Geometry: final body of the model. Coordinates: model frame, mm. A direction names the side the tool comes from. Give positions to 0.01 mm unless a question says otherwise; leave off trailing zeros. Loops run counter-clockwise (first coordinate to the right, second up) from the corner with the lowest first, then second, coordinate; pieces in that order, holes last. Notation, with made-up numbers: (56, 46) -> (67, 46) arc R25 cw to (67, 64) -> close; hole circle Ø7 at (31.25, 61.25). An arc over 180 degrees is marked (long way). Answer in a Markdown table with one row per item. Add a question column.
1) Access query for faces 1 (the cylindrical face through (0.32, 21.08, -13.44)), 2 (the flat face through (-9, -70, 0)), 3 (the flat face through (-20, -77, 0)), 4 (the flat face through (-15, 0, 55)), 5 (the flat face through (0, 18, 58)). Directions: +Z, -Z, +X, -X, +Y, -Y. A direction counts if a zero-diameter tool reaches every point of the face in a straight line with its end or side. Return the directions, or none.
2) Draft query along Z for faces 6 (the flat face through (-23, 5.9, 11.5)), 7 (the flat face through (15, 0, 55)), 8 (the cylindrical face through (37.13, -134.84, -12.92)). Return one class per face: +Z half, -Z half, draft (parallel to the pull), parting line (faces both ways), or undercut.
3) First-contact query: P1, Ø3, axis at x = -10, z = 22.5, coming from the +Y side; P2, Ø11, axis at y = -4.5, z = 44.5, coming from the -X side; P3, Ø10, axis at x = 33, y = -93, coming from the +Z side; P4, Ø19, axis at y = -110, z = 0, coming from the -X side. Flat tips, straight axial feed; report the tip coordinate or a pass-through.
4) Line query: line 1 (X direction, y = -111.5, z = 19); line 2 (Z direction, x = -10.25, y = -110); line 3 (Z direction, x = -8, y = -15). Output: solid intervals per line, ascending. Write a range as from..to.
5) Section query A-A (z = 0). Give the number of separate pieces and of enclosed holes in the cut face, plus the area to 3 significant figures.
6) Section query B-B (x = -2). Return the cut outline in (y, z).
7) Section query D-D (z = 90.5). Return the cut outline in (x, y), plus the area to 3 significant figures.
8) Section query C-C (y = -110). Return the cut outline in (x, z).
```python
from build123d import *

# Parameters (mm, degrees)
SKETCH1_R               = 25
SKETCH1_R_2             = 12.5
BOSS_EXTRUDE1_DEPTH     = 23
BOSS_EXTRUDE3_START     = 20
BOSS_EXTRUDE3_DEPTH     = 18
SKETCH5_R               = 28
SKETCH5_R_2             = 16
BOSS_EXTRUDE4_DEPTH     = 35
BOSS_EXTRUDE5_DEPTH     = 31
CUT_EXTRUDE2_DEPTH      = 155.819249449
CUT_EXTRUDE2_DEPTH_BACK = 155.819249449
SKETCH6_W               = 34
SKETCH6_H               = 70
SKETCH8_R               = 18
SKETCH8_R_2             = 7.5
BOSS_EXTRUDE6_DEPTH     = 24
BOSS_EXTRUDE7_DEPTH     = 21
BOSS_EXTRUDE8_DEPTH     = 9
CUT_EXTRUDE4_DEPTH      = 193.512337267
CUT_EXTRUDE4_DEPTH_BACK = 193.512337267
SKETCH10_W              = 18
SKETCH10_H              = 50


with BuildPart() as part:
    # Sketch1 → Boss-Extrude1 (new, symmetric)
    with BuildSketch(Plane(origin=(0, 0, 0), x_dir=(0, 0, -1), z_dir=(1, 0, 0))):
        Circle(SKETCH1_R)
        Circle(SKETCH1_R_2, mode=Mode.SUBTRACT)
    extrude(amount=BOSS_EXTRUDE1_DEPTH, both=True)

    # Sketch4 → Boss-Extrude3 (add)
    with BuildSketch(Plane(origin=(0, 0, 0), x_dir=(0, 0, -1), z_dir=(1, 0, 0)).offset(BOSS_EXTRUDE3_START)):
        with BuildLine():
            Line((-25, 0), (-25, -70))
            Line((-25, -70), (25, -70))
            Line((25, -70), (25, 0))
            ThreePointArc((25, 0), (0, -25), (-25, 0))
        make_face()
    extrude(amount=-BOSS_EXTRUDE3_DEPTH)



with BuildPart() as body_2:
    # Sketch5 → Boss-Extrude4 (new, symmetric)
    with BuildSketch(Plane(origin=(11, 0, 0), x_dir=(0, 0, -1), z_dir=(1, 0, 0))):
        with Locations((0, -110)):
            Circle(SKETCH5_R)
        with Locations((0, -110)):
            Circle(SKETCH5_R_2, mode=Mode.SUBTRACT)
    extrude(amount=BOSS_EXTRUDE4_DEPTH, both=True)


with BuildPart() as part_1:
    add(part.part)

    add(body_2.part)  # Boss-Extrude5 merges body 2
    # Sketch5_4 → Boss-Extrude5 (add, symmetric)
    with BuildSketch(Plane(origin=(11, 0, 0), x_dir=(0, 0, -1), z_dir=(1, 0, 0))):
        with BuildLine():
            Line((0, -70), (-25, -70))
            Line((-25, -70), (-25, -97.390479787))
            ThreePointArc((-25, -97.390479787), (-14.678784589, -86.156064021), (0, -82))
            Line((0, -82), (0, -70))
        make_face()
        with BuildLine():
            Line((25, -70), (0, -70))
            Line((0, -70), (0, -82))
            ThreePointArc((0, -82), (14.678784589, -86.156064021), (25, -97.390479787))
            Line((25, -97.390479787), (25, -70))
        make_face()
    extrude(amount=BOSS_EXTRUDE5_DEPTH, both=True)

    # Sketch6 → Cut-Extrude2 (cut, two sides: drawn at the far end of the back side and taken through both)
    with BuildSketch(Plane.XY.offset(25).offset(-CUT_EXTRUDE2_DEPTH_BACK)):
        with Locations((11, -117)):
            Rectangle(SKETCH6_W, SKETCH6_H)
    extrude(amount=CUT_EXTRUDE2_DEPTH + CUT_EXTRUDE2_DEPTH_BACK, mode=Mode.SUBTRACT)



with BuildPart() as body_2_2:
    # Sketch8 → Boss-Extrude6 (new, symmetric)
    with BuildSketch(Plane(origin=(0, 0, 0), x_dir=(0, 0, -1), z_dir=(1, 0, 0))):
        with Locations((-85, 0)):
            Circle(SKETCH8_R)
        with Locations((-85, 0)):
            Circle(SKETCH8_R_2, mode=Mode.SUBTRACT)
    extrude(amount=BOSS_EXTRUDE6_DEPTH, both=True)

    # Sketch9 → Boss-Extrude7 (add, symmetric)
    with BuildSketch(Plane(origin=(0, 0, 0), x_dir=(0, 0, -1), z_dir=(1, 0, 0))):
        with BuildLine():
            Line((-55, 18), (-85, 18))
            ThreePointArc((-85, 18), (-67, 0), (-85, -18))
            Line((-85, -18), (-55, -18))
            Line((-55, -18), (-55, 18))
        make_face()
    extrude(amount=BOSS_EXTRUDE7_DEPTH, both=True)


with BuildPart() as part_2:
    add(part_1.part)

    add(body_2_2.part)  # Boss-Extrude8 merges body 2 2
    # Sketch9_3 → Boss-Extrude8 (add, symmetric)
    with BuildSketch(Plane(origin=(0, 0, 0), x_dir=(0, 0, -1), z_dir=(1, 0, 0))):
        with BuildLine():
            Line((-17.349351573, 18), (-55, 18))
            Line((-55, 18), (-55, -18))
            Line((-55, -18), (-25, -18))
            Line((-25, -18), (-25, 0))
            ThreePointArc((-25, 0), (-23.007974588, 9.779218033), (-17.349351573, 18))
        make_face()
    extrude(amount=BOSS_EXTRUDE8_DEPTH, both=True)

    # Sketch10 → Cut-Extrude4 (cut, two sides: drawn at the far end of the back side and taken through both)
    with BuildSketch(Plane(origin=(0, 18, 0), x_dir=(1, 0, 0), z_dir=(0, 1, 0)).offset(-CUT_EXTRUDE4_DEPTH_BACK)):
        with Locations((0, -92)):
            Rectangle(SKETCH10_W, SKETCH10_H)
    extrude(amount=CUT_EXTRUDE4_DEPTH + CUT_EXTRUDE4_DEPTH_BACK, mode=Mode.SUBTRACT)


solid = part_2.part
```
Evaluation:
| question | item | result |
|---|---|---|
| 1 | face 1 | none |
| 1 | face 2 | +Z, -Z, -X |
| 1 | face 3 | -X |
| 1 | face 4 | -X, +Y, -Y |
| 1 | face 5 | +Z, +X, -X, +Y |
| 2 | face 6 | draft |
| 2 | face 7 | undercut |
| 2 | face 8 | parting line |
| 3 | P1 | y = 18 |
| 3 | P2 | x = -9 |
| 3 | P3 | z = 25.3 |
| 3 | P4 | through |
| 4 | line 1 | -24..-6, 28..46 |
| 4 | line 2 | -28..-16, 16..28 |
| 4 | line 3 | -20..20, 25..67 |
| 5 | separate pieces | 4 |
| 5 | enclosed holes | 0 |
| 5 | area | 3,570 mm² |
| 6 | outline | (-82, -25) -> (-70, -25) -> (-70, 25) -> (-82, 25) -> close; (-18, 25) -> (0, 25) arc R25 ccw (long way) to (18, 17.35) -> (18, 67) -> (-18, 67) -> close; hole circle Ø25 at (0, 0) |
| 7 | outline | (-24, -17.14) -> (-9, -17.14) -> (-9, -5.1) -> (-24, -5.1) -> close; (-24, 5.1) -> (-9, 5.1) -> (-9, 17.14) -> (-24, 17.14) -> close; (9, -17.14) -> (24, -17.14) -> (24, -5.1) -> (9, -5.1) -> close; (9, 5.1) -> (24, 5.1) -> (24, 17.14) -> (9, 17.14) -> close |
| 7 | area | 722 mm² |
| 8 | outline | (-24, -28) -> (-6, -28) -> (-6, -16) -> (-24, -16) -> close; (-24, 16) -> (-6, 16) -> (-6, 28) -> (-24, 28) -> close; (28, -28) -> (46, -28) -> (46, -16) -> (28, -16) -> close; (28, 16) -> (46, 16) -> (46, 28) -> (28, 28) -> close |
